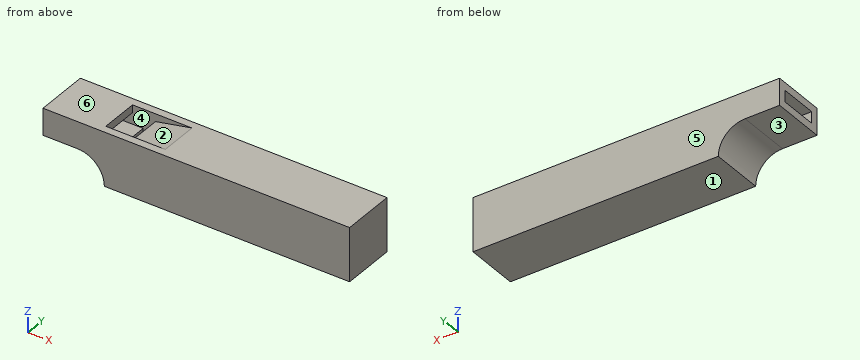
```python
from build123d import *

# Parameters (mm, degrees)
F1_DEPTH = 2
F2_W     = 15
F2_H     = 2
F3_DEPTH = 5


with BuildPart() as f1:
    # F0 (on Front) → F1 (new body)
    with BuildSketch(Plane.XZ):
        with BuildLine():
            ThreePointArc((9, 7), (13.9497474683, 4.9497474683), (16, 0))
            Line((16, 0), (80, 0))
            Line((80, 0), (80, 14))
            Line((80, 14), (0, 14))
            Line((0, 14), (0, 7))
            Line((0, 7), (9, 7))
        make_face()
    extrude(amount=F1_DEPTH)

    # F2 (on face) → F3 (join)
    with BuildSketch(Plane.XZ.offset(2)):
        with BuildLine():
            Line((17.7749643874, 9), (0, 9))
            Line((0, 9), (0, 7))
            Line((0, 7), (9, 7))
            ThreePointArc((9, 7), (13.9497474683, 4.9497474683), (16, 0))
            Line((16, 0), (80, 0))
            Line((80, 0), (80, 14))
            Line((80, 14), (30.5, 14))
            Line((30.5, 14), (21, 12))
            Line((21, 12), (78, 12))
            Line((78, 12), (78, 2))
            Line((78, 2), (17.7749643874, 2))
            Line((17.7749643874, 2), (17.7749643874, 9))
        make_face()
        with Locations((7.5, 13)):
            Rectangle(F2_W, F2_H)
    extrude(amount=F3_DEPTH)

    # F4: F1 across face


with BuildPart() as f1_1:
    add(f1.part)
    add(f1.part.mirror(Plane(origin=(45.1805632689, -7, 6.6042722169), x_dir=(1, 0, 0), z_dir=(0, -1, 0))))


solid = f1_1.part
```
For this review, take the finished solid that the model builds, in its own axes (mm). Face numbers are marked on the shaded views. A direction names the side the tool comes from. Round coordinates to 2 decimals unless told otherwise and drop trailing zeros. Write each loop counter-clockwise with the first axis right and the second up, starting at its lowest first coordinate (ties: lowest second). Pieces come first, ordered by that corner, then holes. Notation, with made-up numbers: (60, 80) - (90, 80) arc R21 ccw to (90, 101) - close; hole circle Ø10 at (24, -25.5). An arc over 180 degrees is marked (long way). Put each result on its own line as item: value.
Q1. We need section D-D (x = 26). Give the boundary of the cut face in (y, z).
Solved:
outline: (-14, 0) - (0, 0) - (0, 14) - (-2, 14) - (-2, 13.05) - (-12, 13.05) - (-12, 14) - (-14, 14) - close; hole (-12, 2) - (-2, 2) - (-2, 12) - (-12, 12) - close
Q2. We need section A-A (x = 45). Give the boundary of the cut face in (y, z), and give its area (3 significant figures).
Solved:
outline: (-14, 0) - (0, 0) - (0, 14) - (-14, 14) - close; hole (-12, 2) - (-2, 2) - (-2, 12) - (-12, 12) - close
area: 96.0 mm2
Q3. Insertion check: pin 1 Ø2.5 at (x, y) = (4.5, -4) entering from -Z; pin 2 Ø5 at (y, z) = (-11, 11) entering from -X; pin 3 Ø5 at (x, y) = (10, -7.5) entering from -Z. Each pin has a flat end and moves straight along its axis. Give the tip position at first contact, or say it passes through.
Solved:
pin 1: stops at z = 7
pin 2: stops at x = 0
pin 3: stops at z = 6.06
Q4. Wall thickness on probe 1 along X at (y, z) = (-11.5, 8.25); probe 2 along Y at (x, z) = (37, 3); probe 3 along Z at (x, y) = (61, -5.5): over which ranges is each line inside the solid? List them lowest first.
Solved:
probe 1: x = 0 to 17.77, 78 to 80
probe 2: y = -14 to -12, -2 to 0
probe 3: z = 0 to 2, 12 to 14
Q5. Mouldability with a two-part tool opening along Z and no side actions: class the marked faces 4, 5 and 6 as released by +Z, released by -Z, zero draft, split by the parting line, or undercut.
Solved:
face 4: undercut
face 5: zero draft
face 6: released by +Z
Q6. Machinability: for the marked faces 1, 2 and 3, which of the approach directions +Z, -Z, +X, -X, +Y, -Y give a long, thin tool a straight path to every point of the face, cutting with its end or side? Answer none if there is none.
Solved:
face 1: -Z, +X, -X, +Y, -Y
face 2: +Z
face 3: -Z, -X, +Y, -Y
Q7. We need section B-B (z = 7.75). Give the boundary of the cut face in (x, y).
Solved:
outline: (0, -14) - (80, -14) - (80, 0) - (0, 0) - close; hole (17.77, -12) - (78, -12) - (78, -2) - (17.77, -2) - close
Q8. We need section C-C (y = -8.75). Give the boundary of the cut face in (x, z).
Solved:
outline: (0, 7) - (9, 7) arc R7 cw to (16, 0) - (80, 0) - (80, 14) - (30.5, 14) - (21, 12) - (78, 12) - (78, 2) - (17.77, 2) - (17.77, 9) - (0, 9) - close; (0, 12) - (15, 12) - (15, 14) - (0, 14) - close
